For this review, take the finished solid that the model builds, in its own axes (mm). A direction names the side the tool comes from. Round coordinates to 2 decimals unless told otherwise and drop trailing zeros. Write each loop counter-clockwise with the first axis right and the second up, starting at its lowest first coordinate (ties: lowest second). Pieces come first, ordered by that corner, then holes. Notation, with made-up numbers: M 12,-37.75 L 57,-37.75 A11 ccw 57,-25.75 Z; hole C -4,53.5 d5. An arc over 180 degrees is marked long. Use one line per item in the form item = value. Start each with the question number.
Item 1: For faces 5 (the flat face through (0, 0, 7)), 6 (the flat face through (-4, 2, 9)), 7 (the cylindrical face through (4.37, 11.07, 18.1)), list the 3-axis set-ups (+Z, -Z, +X, -X, +Y, -Y) from which the entire face can be reached by the end or side of a thin tool; tool diameter is ignored.
Item 2: Add section C-C (y = 9.5). State the section outline as (x, z) points.
Item 3: Add section B-B (y = 1.5). State the section outline as (x, z) points, and give its area (3 significant figures).
Item 4: For P1, Ø1.5, axis at x = 0, z = 2.5, coming from the +Y side; P2, Ø4, axis at x = -1.5, y = -1.5, coming from the -Z side; P3, Ø4, axis at y = -1.5, z = 10.5, coming from the -X side; P4, Ø4, axis at y = 9.5, z = 12.5, coming from the -X side, all flat-tipped, find the tip position at first contact; note any pin that passes through.
Item 5: For line 1 (X direction, y = 3.8, z = 0); line 2 (Y direction, x = -3.25, z = 12); line 3 (Y direction, x = 0.25, z = 20.5), list the stretches that pass through material, from the lowest coordinate up. Write a range as [from, to].
Item 6: Add section D-D (y = 5.75). State the section outline as (x, z) points, and give its area (3 significant figures).
Item 7: Add section A-A (z = 0). State the section outline as (x, y) points.
Item 8: Draft analysis for pull direction Z (two halves, no side actions). For faces 1 (the flat face through (0, 5, 7)), 2 (the cylindrical face through (1.528, 10.483, 19.655)), 3 (the cylindrical face through (3.033, -3.412, 18.786)), 4 (the flat face through (2.51, 2.64, 22.015)), state which applies: released by +Z, released by -Z, zero draft, split by the parting line, or undercut.
from build123d import *

# Parameters (mm, degrees)
SKETCH1_R           = 2.147718393
BOSS_EXTRUDE1_DEPTH = 5
SKETCH2_W           = 10
SKETCH2_H           = 20
BOSS_EXTRUDE2_DEPTH = 5
SKETCH3_R           = 2
CUT_EXTRUDE1_DEPTH  = 5
FILLET1_R           = 5


with BuildPart() as part:
    # Sketch1 → Boss-Extrude1 (new body)
    with BuildSketch(Plane(origin=(0, 0, 0), x_dir=(1, 0, 0), z_dir=(0, 1, 0))):
        with BuildLine():
            Line((-4, -20), (4, -15.381197846))
            Line((4, -15.381197846), (4, -5))
            Line((4, -5), (4, 1.25))
            ThreePointArc((4, 1.25), (2.901650429, 3.901650429), (0.25, 5))
            Line((0.25, 5), (-0.25, 5))
            ThreePointArc((-0.25, 5), (-2.901650429, 3.901650429), (-4, 1.25))
            Line((-4, 1.25), (-4, -5))
            Line((-4, -5), (-4, -20))
        make_face()
        with Locations(Location((0, 0, 0), (0, 0, 270))):
            Circle(SKETCH1_R, mode=Mode.SUBTRACT)
    extrude(amount=BOSS_EXTRUDE1_DEPTH)

    # Sketch2 → Boss-Extrude2 (add)
    with BuildSketch(Plane(origin=(7.660254038, 0, 13.267949192), x_dir=(0.8660254037844382, 0, -0.500000000000001), z_dir=(0.5000000000000009, 0, 0.866025403784438))):
        with Locations((-8.764101615, 2.5)):
            Rectangle(SKETCH2_W, SKETCH2_H)
    extrude(amount=BOSS_EXTRUDE2_DEPTH)

    # Sketch3 → Cut-Extrude1 (cut)
    with BuildSketch(Plane(origin=(7.660254038, 0, 13.267949192), x_dir=(-0.8660254037844382, 0, 0.5000000000000009), z_dir=(-0.5000000000000009, 0, -0.8660254037844383))):
        with Locations((8.764101615, -3.5)):
            Circle(SKETCH3_R)
        with Locations((8.764101615, 8.5)):
            Circle(SKETCH3_R)
    extrude(amount=-CUT_EXTRUDE1_DEPTH, mode=Mode.SUBTRACT)

    # Fillet1
    fillet1_edges = [part.edges().sort_by_distance(p)[0] for p in [
        (5.650446417, 12.5, 17.315063509),
        (-3.009807621, 12.5, 22.315063509),
        (5.650446417, -7.5, 17.315063509),
        (-3.009807621, -7.5, 22.315063509),
    ]]
    fillet(fillet1_edges, radius=FILLET1_R - 0.0001)  # a hair under: the kernel refuses the full size


solid = part.part
Calculated:
q1.face_5 = -Z, -X, -Y
q1.face_6 = -Z, -X, +Y, -Y
q1.face_7 = -Z, +X, +Y
q2.outline = M -3.9,19.94 L -1.43,18.52 L 1.07,22.85 L -1.4,24.27 Z; M 1.57,16.78 L 4.04,15.36 L 6.54,19.69 L 4.07,21.11 Z
q3.outline = M -4.26,20.15 L -4,20 L -4,-1.25 A3.75 ccw -0.25,-5 L 0.25,-5 A3.75 ccw 4,-1.25 L 4,15.38 L 4.4,15.15 L 6.9,19.48 L -1.76,24.48 Z; hole C 0,0 d4.3
q3.area = 211 mm^2
q4.P1 = 5
q4.P2 = -5
q4.P3 = -4
q4.P4 = through
q5.line_1 = [-4, -2.15], [2.15, 4]
q5.line_2 = [0, 5]
q5.line_3 = [-7.34, -5.05], [-1.95, 6.95], [10.05, 12.34]
q6.outline = M -4.26,20.15 L 4.4,15.15 L 6.9,19.48 L -1.76,24.48 Z
q6.area = 50.0 mm^2
q7.outline = M -4,0 L -2.15,0 L -2.15,5 L -4,5 Z; M 2.15,0 L 4,0 L 4,5 L 2.15,5 Z
q8.face_1 = zero draft
q8.face_2 = undercut
q8.face_3 = undercut
q8.face_4 = released by +Z
